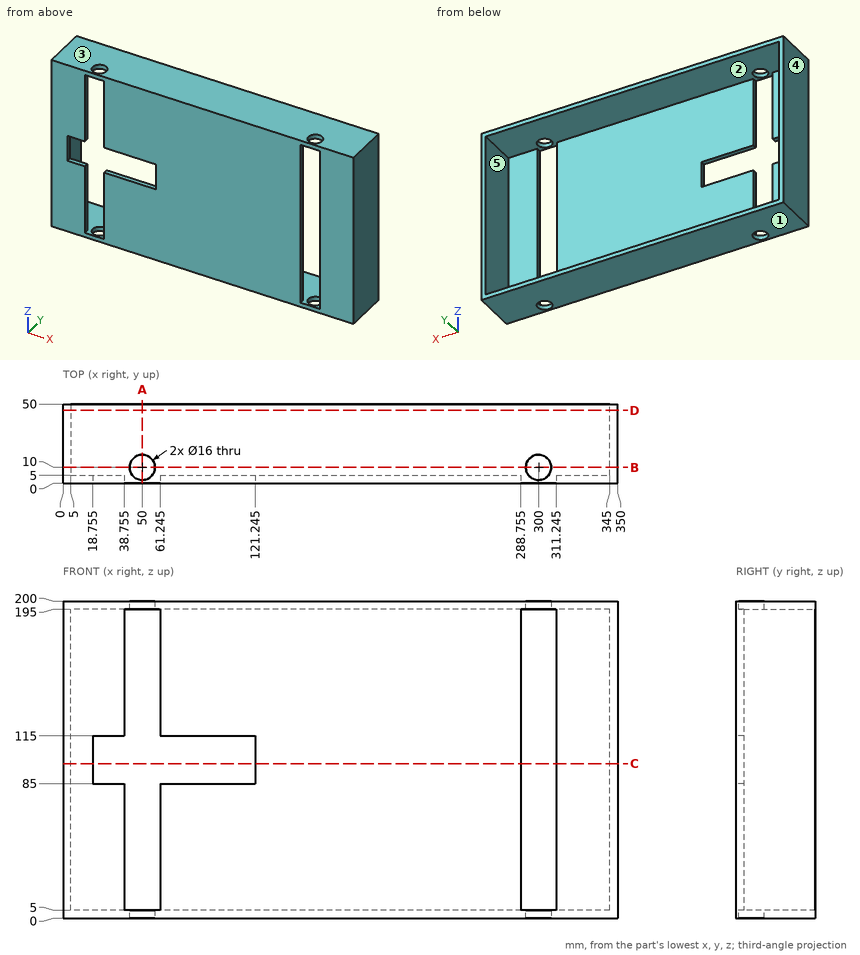
Here's the drawing with two shaded views (mm, measured from the low corner). I have some questions. A direction names the side the tool comes from. Round coordinates to 2 decimals unless told otherwise and drop trailing zeros. Order: outer loops, then holes, each group sorted by start corner. A loop starts at its lowest first (then second) coordinate and runs counter-clockwise, first axis right, second up. Notation, with made-up numbers: (24, 11.25) -> (31, 11.25) arc R8 cw to (31, 15.25) -> close; hole circle Ø4 at (-7, 32.25). An arc over 180 degrees is marked (long way). Write each question's results on one line, items separated by ' | '. Start each with the question number.
Item 1: Please list where these lines run through material, in increasing order: L1, parallel to X at y = 3, z = 129 (3 decimals); L2, parallel to Z at x = 118, y = 24; L3, parallel to X at y = 11, z = 116.5.
Item 2: If we section it at B-B, the plane y = 10: Write out the boundary of the cut face in (x, z).
Item 3: If we section it at A-A, the plane x = 50: Write out the boundary of the cut face in (y, z).
Item 4: Which directions (+Z, -Z, +X, -X, +Y, -Y) give clear straight access to the entire face, cutting with the end or side of a thin tool? Please do the marked faces 1 and 2.
Item 5: If we section it at D-D, the plane y = 46: Write out the boundary of the cut face in (x, z), then the cut area to 3 significant figures.
Item 6: Will these pins go through, and if not, where does the flat tip stop? pin 1 (8 mm diameter, centred on x = 295, z = 40, fed in from -Y); pin 2 (12 mm diameter, centred on x = 91.5, z = 78, fed in from +Y).
Item 7: Thinking about a two-plate mould opening in X: for the marked faces 3, 4 and 5, which applies, +X half, -X half, draft (parallel to the pull), parting line (faces both ways), or undercut?
Item 8: If we section it at C-C, the plane z = 97.5: Write out the boundary of the cut face in (x, y) (3 decimals), then the cut area to 3 significant figures.
Results:
1) L1: x = 0 to 38.755, 61.245 to 288.755, 311.245 to 350 | L2: z = 0 to 5, 195 to 200 | L3: x = 0 to 5, 345 to 350
2) outline: (0, 0) -> (42, 0) -> (42, 5) -> (5, 5) -> (5, 195) -> (42, 195) -> (42, 200) -> (0, 200) -> close; (58, 0) -> (292, 0) -> (292, 5) -> (58, 5) -> close; (58, 195) -> (292, 195) -> (292, 200) -> (58, 200) -> close; (308, 0) -> (350, 0) -> (350, 200) -> (308, 200) -> (308, 195) -> (345, 195) -> (345, 5) -> (308, 5) -> close
3) outline: (0, 0) -> (2, 0) -> (2, 5) -> (0, 5) -> close; (0, 195) -> (2, 195) -> (2, 200) -> (0, 200) -> close; (18, 0) -> (50, 0) -> (50, 5) -> (18, 5) -> close; (18, 195) -> (50, 195) -> (50, 200) -> (18, 200) -> close
4) face 1: -Z, +X, -X, +Y, -Y | face 2: +Y
5) outline: (0, 0) -> (350, 0) -> (350, 200) -> (0, 200) -> close; hole (5, 5) -> (345, 5) -> (345, 195) -> (5, 195) -> close | area: 5,400 mm2
6) pin 1: passes through | pin 2: stops at y = 5
7) face 3: draft | face 4: -X half | face 5: undercut
8) outline: (0, 0) -> (18.755, 0) -> (18.755, 5) -> (5, 5) -> (5, 50) -> (0, 50) -> close; (121.245, 0) -> (288.755, 0) -> (288.755, 5) -> (121.245, 5) -> close; (311.245, 0) -> (350, 0) -> (350, 50) -> (345, 50) -> (345, 5) -> (311.245, 5) -> close | area: 1,580 mm2
